Solid Edge part; units mm, degrees
sketch "Sketch1" plane through (-21.59, -31.75, -17.5119) normal (0, 0, -1) x (0, -1, 0)
  line L0 (56.642, -17.4625) -> (56.642, 17.4625)
  arc A0 (40.767, 33.3375) -> (56.642, 17.4625) centre (40.767, 17.4625) cw
  line L1 (40.767, 33.3375) -> (-40.767, 33.3375)
  arc A1 (-40.767, 33.3375) -> (-56.642, 17.4625) centre (-40.767, 17.4625) ccw
  line L2 (-56.642, 17.4625) -> (-56.642, -17.4625)
  arc A2 (-40.767, -33.3375) -> (-56.642, -17.4625) centre (-40.767, -17.4625) cw
  line L3 (-40.767, -33.3375) -> (40.767, -33.3375)
  arc A3 (40.767, -33.3375) -> (56.642, -17.4625) centre (40.767, -17.4625) ccw
  circle A4 centre (51.2445, 0) radius 2.0955
  circle A5 centre (51.2445, 17.4625) radius 2.0955
  circle A6 centre (47.3092, 26.9819) radius 2.0955
  circle A7 centre (51.2445, -17.4625) radius 2.0955
  circle A8 centre (47.3092, -26.9819) radius 2.0955
  circle A9 centre (-47.3092, 26.9819) radius 2.0955
  circle A10 centre (-51.2445, 17.4625) radius 2.0955
  circle A11 centre (-51.2445, 0) radius 2.0955
  circle A12 centre (-51.2445, -17.4625) radius 2.0955
  circle A13 centre (-47.3092, -26.9819) radius 2.0955
extrude "Protrusion1" add sketch "Sketch1" along normal blind 6.35
extrude "ExtrudedCutout_1" [suppressed]
sketch "Sketch2" plane through (-21.59, -31.75, -17.5119) normal (0, 0, -1) x (0, -1, 0)
  line L0 (42.672, -17.4625) -> (42.672, 17.4625)
  arc A0 (42.672, 17.4625) -> (29.972, 30.1625) centre (29.972, 17.4625) ccw
  line L1 (29.972, 30.1625) -> (-29.972, 30.1625)
  arc A1 (-42.672, 17.4625) -> (-29.972, 30.1625) centre (-29.972, 17.4625) cw
  line L2 (-42.672, 17.4625) -> (-42.672, -17.4625)
  arc A2 (-29.972, -30.1625) -> (-42.672, -17.4625) centre (-29.972, -17.4625) cw
  line L3 (-29.972, -30.1625) -> (29.972, -30.1625)
  arc A3 (42.672, -17.4625) -> (29.972, -30.1625) centre (29.972, -17.4625) cw
sketch "Sketch3" plane through (-21.59, -76.5773, -17.5119) normal (1, 0, 0) x (0, 0.7809, -0.6247)
  line L0 (0.4433, 0.3547) -> (2.9226, 2.3381)
  line L1 (2.0003, 0.9497) -> (2.9226, 2.3381)
  line L2 (0.4433, 0.3547) -> (2.0003, 0.9497)
sweep "SweptCutout_2" cut profiles "Sketch3" path "Sketch2"
sketch "Sketch4" plane through (-21.59, -31.75, -23.8619) normal (0, 0, -1) x (0, -1, 0)
  circle A0 centre (47.3092, 26.9819) radius 3.4925
  circle A1 centre (51.2445, 17.4625) radius 3.4925
  circle A2 centre (51.2445, 0) radius 3.4925
  circle A3 centre (51.2445, -17.4625) radius 3.4925
  circle A4 centre (47.3092, -26.9819) radius 3.4925
  circle A5 centre (-47.3092, -26.9819) radius 3.4925
  circle A6 centre (-51.2445, -17.4625) radius 3.4925
  circle A7 centre (-51.2445, 0) radius 3.4925
  circle A8 centre (-51.2445, 17.4625) radius 3.4925
  circle A9 centre (-47.3092, 26.9819) radius 3.4925
extrude "counter_sink" cut sketch "Sketch4" against normal blind 2.54
sketch "Sketch5" plane through (-21.59, -31.75, -23.8619) normal (0, 0, -1) x (0, -1, 0)
  line L0 (39.37, -30.9245) -> (-39.37, -30.9245)
  line L1 (-39.37, -30.9245) -> (-39.37, -29.4005)
  line L2 (-39.37, -29.4005) -> (39.37, -29.4005)
  line L3 (39.37, -29.4005) -> (39.37, -30.9245)
  line L4 (-39.37, 29.4005) -> (39.37, 29.4005)
  line L5 (39.37, 29.4005) -> (39.37, 30.9245)
  line L6 (39.37, 30.9245) -> (-39.37, 30.9245)
  line L7 (-39.37, 30.9245) -> (-39.37, 29.4005)
extrude "ExtrudedCutout_3" cut sketch "Sketch5" against normal blind 2.286
sketch "Sketch6" plane through (-21.59, -31.75, -17.5119) normal (0, 0, 1) x (-1, 0, 0)
  line L0 (-17.145, 38.1) -> (17.145, 38.1)
  arc A0 (17.145, 38.1) -> (25.4, 29.845) centre (17.145, 29.845) cw
  line L1 (25.4, 29.845) -> (25.4, -29.845)
  arc A1 (25.4, -29.845) -> (17.145, -38.1) centre (17.145, -29.845) cw
  line L2 (17.145, -38.1) -> (-17.145, -38.1)
  arc A2 (-17.145, -38.1) -> (-25.4, -29.845) centre (-17.145, -29.845) cw
  line L3 (-25.4, -29.845) -> (-25.4, 29.845)
  arc A3 (-17.145, 38.1) -> (-25.4, 29.845) centre (-17.145, 29.845) ccw
extrude "thin_the_center_of_the_lid" cut sketch "Sketch6" against normal blind 4.7625
CAD build for the part. Positions are in the model's coordinates, mm. A direction names the side the tool comes from. Round coordinates to 2 decimals unless told otherwise and drop trailing zeros. Order: outer loops, then holes, each group sorted by start corner. A loop starts at its lowest first (then second) coordinate and runs counter-clockwise, first axis right, second up. Notation, with made-up numbers: (40.25, 3.25) -> (89.25, 3.25) arc R14 ccw to (89.25, 21.25) -> close; hole circle Ø9 at (27, -12.75). An arc over 180 degrees is marked (long way). Write item = value, one per line.
(1) Pull direction X, two halves, no side cores. Call faces 4 (the flat face through (4, -32, -17.512)), 5 (the cylindrical face through (-50.15, 20.37, -20.64)), 6 (the conical face through (-48.33, -70.8, -17.93)), 7 (the cylindrical face through (-19.465, -80.223, -22.61)): +X half, -X half, draft (parallel to the pull), parting line (faces both ways), or undercut.
Answers follow:
face_4 = draft
face_5 = -X half
face_6 = undercut
face_7 = undercut
(2) 3-axis set-ups, long thin cutter, end or side, ignore diameter. For faces 1 (the flat face through (11, -36, -17.512)), 2 (the flat face through (-50.99, -31, -23)), 3 (the conical face through (5.15, 7.3, -17.93)): which of +Z, -Z, +X, -X, +Y, -Y reach the whole face in a straight line?
Answers follow:
face_1 = +Z, +X, -X, +Y, -Y
face_2 = -Z
face_3 = +Z
(3) Cut at A-A (x = -21.59). State how many separate pieces and enclosed holes the cut face has, plus the area to 3 significant figures.
Answers follow:
separate_pieces = 3
enclosed_holes = 0
area = 287 mm²
(4) Drill centre lines: L1, parallel to X at y = -6.5, z = -22.75; L2, parallel to Y at x = -21.59, z = -20.45; L3, parallel to X at y = -43, z = -18.75. Where is each one in solid material? Low to high.
Answers follow:
L1 = -54.93 to -52.51, -50.99 to 7.81, 9.33 to 11.75
L2 = -88.39 to -85.09, -80.9 to -69.85, 6.35 to 17.4, 21.59 to 24.89
L3 = -54.93 to -46.99, 3.81 to 11.75
(5) Flat gauge pin, fed straight in: P1, Ø3.5, axis at x = -20.5, y = 19, coming from the -Z side. Where does the tip first touch, or does it go through?
Answers follow:
P1 = -21.32
(6) Cut at B-B (y = -20.5). Write the cut outline in (x, z), plus the area to 3 significant figures.
Answers follow:
outline = (-54.93, -23.86) -> (-52.51, -23.86) -> (-52.51, -21.58) -> (-50.99, -21.58) -> (-50.99, -23.86) -> (7.81, -23.86) -> (7.81, -21.58) -> (9.33, -21.58) -> (9.33, -23.86) -> (11.75, -23.86) -> (11.75, -17.51) -> (10.16, -17.51) -> (8.57, -18.02) -> (6.99, -17.51) -> (3.81, -17.51) -> (3.81, -22.27) -> (-46.99, -22.27) -> (-46.99, -17.51) -> (-50.17, -17.51) -> (-51.75, -18.02) -> (-53.34, -17.51) -> (-54.93, -17.51) -> close
area = 173 mm²
